from build123d import *

# Parameters (mm, degrees)
F0_W      = 96.012
F0_H      = 86.36
F1_DEPTH  = 53.848
F2_T      = -5.08
F4_D      = 6.35
F6_DEPTH  = 25.4
F7_W      = 84.328
F7_H      = 66.04
F8_DEPTH  = 25.4
F9_W      = 53.848
F9_H      = 58.42
F10_DEPTH = 25.4
F11_W     = 85.852
F11_H     = 5.08
F12_DEPTH = 15.24
F13_DEPTH = 10.16
F14_DEPTH = 12.7


# Not quite as in the source:
# - a feature names something its author has since deleted; it is built from what else it names


with BuildPart() as f1:
    # F0 (on Front) → F1 (new body)
    with BuildSketch(Plane.XZ):
        with Locations((48.006, 43.18)):
            Rectangle(F0_W, F0_H)
    extrude(amount=F1_DEPTH)

    # F2
    f2_openings = [f1.faces().sort_by_distance(p)[0] for p in [
        (48.006, -26.924, 86.36),
        (48.006, 0, 43.18),
    ]]
    offset(amount=F2_T, openings=f2_openings)

    # F4 (through all)
    with Locations(Plane(origin=(0, 0, 0), x_dir=(1, 0, 0), z_dir=(0, 0, -1))):
        with Locations((17.018, 30.7086)):
            Hole(F4_D / 2)

    # F5 (on face) → F6 (cut)
    with BuildSketch(Plane(origin=(0, 0, 0), x_dir=(1, 0, 0), z_dir=(0, 0, -1))):
        with BuildLine():
            Line((76.962, 25.908), (46.482, 25.908))
            ThreePointArc((46.482, 25.908), (44.6859487758, 25.1640512242), (43.942, 23.368))
            Line((43.942, 23.368), (43.942, 13.97))
            ThreePointArc((43.942, 13.97), (44.6859487758, 12.1739487758), (46.482, 11.43))
            Line((46.482, 11.43), (76.962, 11.43))
            ThreePointArc((76.962, 11.43), (78.7580512242, 12.1739487758), (79.502, 13.97))
            Line((79.502, 13.97), (79.502, 23.368))
            ThreePointArc((79.502, 23.368), (78.7580512242, 25.1640512242), (76.962, 25.908))
        make_face()
    extrude(amount=-F6_DEPTH, mode=Mode.SUBTRACT)

    # F7 (on face) → F8 (cut)
    with BuildSketch(Plane.XZ.offset(53.848)):
        with Locations((47.498, 53.34)):
            Rectangle(F7_W, F7_H)
    extrude(amount=-F8_DEPTH, mode=Mode.SUBTRACT)

    # F9 (on face) → F10 (cut)
    with BuildSketch(Plane(origin=(0, 0, 0), x_dir=(0, -1, 0), z_dir=(-1, 0, 0))):
        with Locations((26.924, 57.15)):
            Rectangle(F9_W, F9_H)
    extrude(amount=-F10_DEPTH, mode=Mode.SUBTRACT)

    # F11 (on face) → F12 (join)
    with BuildSketch(Plane.XY.offset(5.08)):
        with Locations((48.006, -2.54)):
            Rectangle(F11_W, F11_H)
    extrude(amount=F12_DEPTH)

    # F13 (add): a face of the model
    f13_faces = [f1.faces().sort_by_distance(p)[0] for p in [
        (5.334, -51.308, 24.13),
    ]]
    extrude(f13_faces, amount=F13_DEPTH)

    # F14 (add): a face of the model
    f14_faces = [f1.faces().sort_by_distance(p)[0] for p in [
        (89.662, -51.308, 53.34),
    ]]
    extrude(f14_faces, amount=F14_DEPTH)


solid = f1.part
Verification items for the finished model (mm, model axes). A direction names the side the tool comes from. Give positions to 0.01 mm unless a question says otherwise; leave off trailing zeros. Write each loop counter-clockwise with the first axis right and the second up, starting at its lowest first coordinate (ties: lowest second). Pieces come first, ordered by that corner, then holes. Notation, with made-up numbers: (16.25, -32.5) - (40.25, -32.5) arc R21 cw to (40.25, -16.5) - close; hole circle Ø9 at (15, 52). An arc over 180 degrees is marked (long way). Answer as CSV lines item,"result". Start each with the question number.
1. Sectioned sample at D-D (x = 29.5). Record the boundary of the cut face in (y, z), then the cut area to 3 significant figures.
2. Set-up check for faces 5 (the face through (62, -11.43, 3)), 6 (the face through (15.494, -51, 24)), 7 (the face through (91.5, -33, 86.36)): record each of +Z, -Z, +X, -X, +Y, -Y from which the full face is reachable in a straight line by a thin tool's end or side.
3. Sectioned sample at A-A (x = 58). Record the boundary of the cut face in (y, z).
4. Thickness scan on line 1 (Y direction, x = 51.5, z = 10); line 2 (X direction, y = -14, z = 27.5); line 3 (X direction, y = -51, z = 23). Record the ranges inside material, lowest first.
5. Sectioned sample at B-B (z = 23.5). Record the boundary of the cut face in (x, y).
6. Sectioned sample at C-C (y = -41.5). Record the boundary of the cut face in (x, z).
7. Depth check by flat-ended pin: pin 1 (4 mm diameter, centred on y = -52, z = 58, fed in from -X); pin 2 (5.5 mm diameter, centred on x = 50.5, y = -51, fed in from +Z); pin 3 (3 mm diameter, centred on x = 85.5, z = 44.5, fed in from +Y). Enter the tip coordinate at first touch or a pass-through.
8. Draft check along Y on faces 1 (the face through (4, -33, 27.94)), 2 (the face through (47, -5.08, 13)), 3 (the face through (51, 0, 15)), 4 (the face through (78.78, -25.14, 2.5)). Enter one of: pulls with the +Y half, pulls with the -Y half, needs draft (parallel to the pull), parting line crosses it, or undercut.
Derived:
1,outline,"(-53.85, 0) - (0, 0) - (0, 20.32) - (-5.08, 20.32) - (-5.08, 5.08) - (-48.77, 5.08) - (-48.77, 20.32) - (-53.85, 20.32) - close"
1,area,"428 mm²"
2,face 5,"+Z, -Z"
2,face 6,"+Z, +Y, -Y"
2,face 7,"+Z, +X, -X, +Y, -Y"
3,outline,"(-53.85, 0) - (-25.91, 0) - (-25.91, 5.08) - (-48.77, 5.08) - (-48.77, 20.32) - (-53.85, 20.32) - close; (-11.43, 0) - (0, 0) - (0, 20.32) - (-5.08, 20.32) - (-5.08, 5.08) - (-11.43, 5.08) - close"
4,line 1,"-53.85 to -48.77, -5.08 to 0"
4,line 2,"0 to 5.08, 90.93 to 96.01"
4,line 3,"0 to 15.49, 76.96 to 96.01"
5,outline,"(0, -53.85) - (15.49, -53.85) - (15.49, -48.77) - (5.08, -48.77) - (5.08, 0) - (0, 0) - close; (76.96, -53.85) - (96.01, -53.85) - (96.01, 0) - (90.93, 0) - (90.93, -48.77) - (76.96, -48.77) - close"
6,outline,"(0, 0) - (96.01, 0) - (96.01, 86.36) - (90.93, 86.36) - (90.93, 5.08) - (5.08, 5.08) - (5.08, 27.94) - (0, 27.94) - close"
7,pin 1,"x = 76.96"
7,pin 2,"z = 20.32"
7,pin 3,"y = -48.77"
8,face 1,"needs draft"
8,face 2,"undercut"
8,face 3,"pulls with the +Y half"
8,face 4,"undercut"
